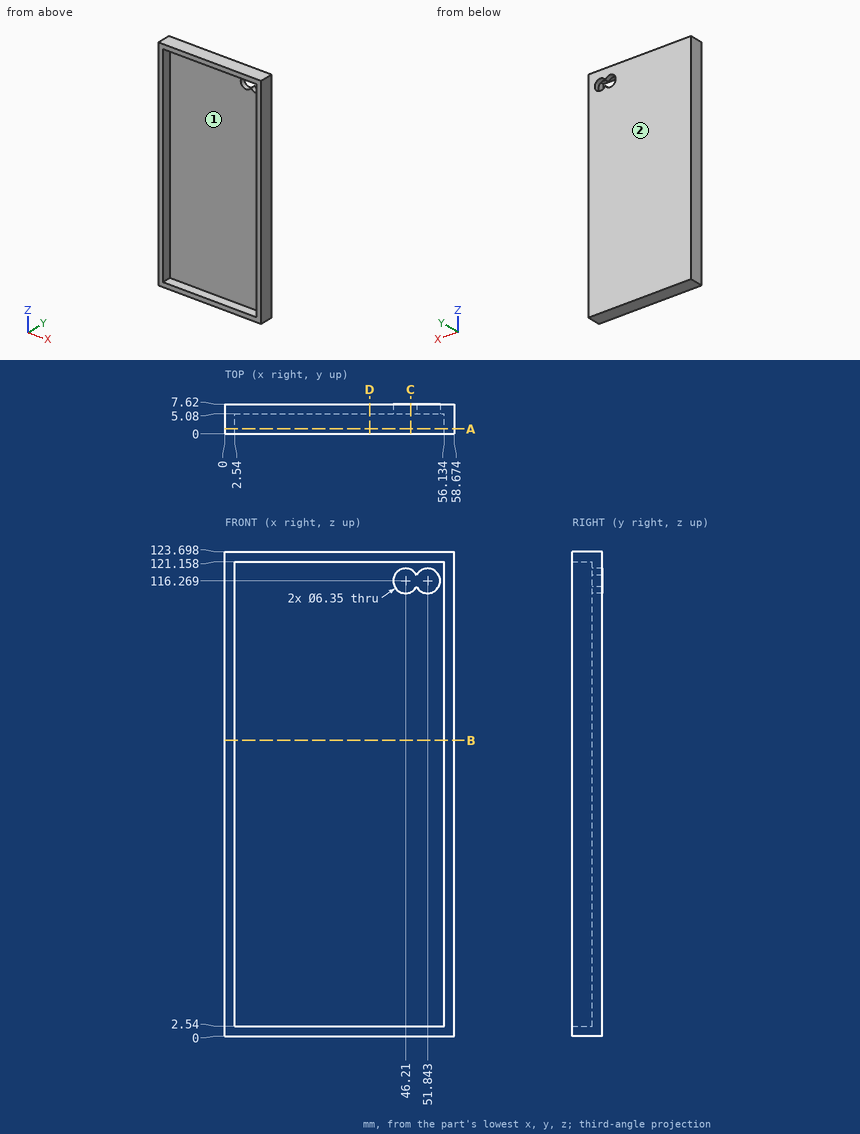
Source: three-view drawing plus pictorial views. Frame: mm from the lowest corner of the part. Round coordinates to 2 decimals unless told otherwise and drop trailing zeros. Loops run counter-clockwise (first coordinate to the right, second up) from the corner with the lowest first, then second, coordinate; pieces in that order, holes last.
Q1. Section B-B, the plane z = 75.5. Return loops of the section in (x, y), plus the area to 3 significant figures.
Q2. Ray query, line 1 (X direction, y = 3.75, z = 13); line 2 (Z direction, x = 31, y = 1); line 3 (Y direction, x = 27.5, z = 36). Return the intervals inside material, ascending.
Q3. Section C-C, the plane x = 47.5. Return loops of the section in (y, z).
Q4. First-contact query: P1, Ø10, axis at x = 7.5, z = 35.5, coming from the -Y side; P2, Ø4, axis at x = 26, z = 89, coming from the -Y side. Flat tips, straight axial feed; report the tip coordinate or a pass-through.
Q5. Section A-A, the plane y = 1.25. Return loops of the section in (x, z).
Q6. Mould query, pull axis Z, two halves, no side actions, for the marked faces 1 and 2. Classes: pulls with the +Z half, pulls with the -Z half, needs draft (parallel to the pull), parting line crosses it, or undercut.
Q7. Section D-D, the plane x = 37. Return loops of the section in (y, z), plus the area to 3 significant figures.
Solutions:
1. outline: (0, 0) - (2.54, 0) - (2.54, 5.08) - (56.13, 5.08) - (56.13, 0) - (58.67, 0) - (58.67, 7.62) - (0, 7.62) - close
1. area: 175 mm2
2. line 1: x = 0 to 2.54, 56.13 to 58.67
2. line 2: z = 0 to 2.54, 121.16 to 123.7
2. line 3: y = 5.08 to 7.62
3. outline: (0, 0) - (7.62, 0) - (7.62, 113.37) - (5.08, 113.37) - (5.08, 2.54) - (0, 2.54) - close; (0, 121.16) - (5.08, 121.16) - (5.08, 119.17) - (7.62, 119.17) - (7.62, 123.7) - (0, 123.7) - close
4. P1: stops at y = 0
4. P2: stops at y = 5.08
5. outline: (0, 0) - (58.67, 0) - (58.67, 123.7) - (0, 123.7) - close; hole (2.54, 2.54) - (56.13, 2.54) - (56.13, 121.16) - (2.54, 121.16) - close
6. face 1: undercut
6. face 2: needs draft
7. outline: (0, 0) - (7.62, 0) - (7.62, 123.7) - (0, 123.7) - (0, 121.16) - (5.08, 121.16) - (5.08, 2.54) - (0, 2.54) - close
7. area: 340 mm2
